```python
from build123d import *

# Parameters (mm, degrees)
F1_DEPTH  = 8
F2_W      = 15
F2_H      = 12
F2_W_2    = 4
F2_W_3    = 22
F2_W_4    = 0.5
F3_DEPTH  = 2
F4_DEPTH  = 3
F2_W_5    = 12
F2_W_6    = 2
F5_DEPTH  = 5
F6_DEPTH  = 4
F8_W      = 36.5
F8_H      = 1
F7_W      = 36.5
F7_H      = 1
F9_DEPTH  = 1
F2_H_2    = 1.5
F10_DEPTH = 3
F11_DEPTH = 2
F12_DEPTH = 2
F13_DEPTH = 3


with BuildPart() as f1:
    # F0 (on Top) → F1 (new body)
    with BuildSketch(Plane.XY):
        Polygon((-40, -7.5), (-25, -17.5), (25, -17.5), (40, -7.5), (85, -7.5), (85, 7.5), (40, 7.5), (25, 17.5), (-25, 17.5), (-40, 7.5), (-85, 7.5), (-85, -7.5), align=None)
    extrude(amount=F1_DEPTH)

    # F2 (on face) → F3 (cut)
    with BuildSketch(Plane.XY.offset(8)):
        with Locations((-77.5, 0)):
            Rectangle(F2_W, F2_H)
        with Locations((-68, 0)):
            Rectangle(F2_W_2, F2_H)
        with Locations((-55, 0)):
            Rectangle(F2_W_3, F2_H)
        with Locations((-43.75, 0)):
            Rectangle(F2_W_4, F2_H)
        with Locations((77.5, 0)):
            Rectangle(F2_W, F2_H)
        with Locations((68, 0)):
            Rectangle(F2_W_2, F2_H)
        with Locations((55, 0)):
            Rectangle(F2_W_3, F2_H)
        with Locations((43.75, 0)):
            Rectangle(F2_W_4, F2_H)
    extrude(amount=-F3_DEPTH, mode=Mode.SUBTRACT)

    # F2 (on face) → F4 (cut)
    with BuildSketch(Plane.XY.offset(8)):
        with Locations((-36, 0)):
            Rectangle(F2_W, F2_H)
        with Locations((36, 0)):
            Rectangle(F2_W, F2_H)
    extrude(amount=-F4_DEPTH, mode=Mode.SUBTRACT)

    # F2 (on face) → F5 (cut)
    with BuildSketch(Plane.XY.offset(8)):
        with Locations((-22.5, 0)):
            Rectangle(F2_W_5, F2_H)
        with Locations((-15.5, 0)):
            Rectangle(F2_W_6, F2_H)
        with Locations((15.5, 0)):
            Rectangle(F2_W_6, F2_H)
        with Locations((22.5, 0)):
            Rectangle(F2_W_5, F2_H)
    extrude(amount=-F5_DEPTH, mode=Mode.SUBTRACT)

    # F2 (on face) → F6 (cut)
    with BuildSketch(Plane.XY.offset(8)):
        Polygon((16.5, 11), (-16.5, 11), (-16.5, 6), (-14.5, 6), (-14.5, -6), (-16.5, -6), (-16.5, -11), (16.5, -11), (16.5, -6), (14.5, -6), (14.5, 6), (16.5, 6), align=None)
    extrude(amount=-F6_DEPTH, mode=Mode.SUBTRACT)

    # F8 (on face) + F7 (on face) → F9 (cut)
    with BuildSketch(Plane.XY.offset(6)):
        with Locations((61.75, 0)):
            Rectangle(F8_W, F8_H)
    with BuildSketch(Plane.XY.offset(6)):
        with Locations((-61.75, 0)):
            Rectangle(F7_W, F7_H)
    extrude(amount=-F9_DEPTH, mode=Mode.SUBTRACT)

    # F2 (on face) → F10 (cut)
    with BuildSketch(Plane.XY.offset(8)):
        with Locations((-77.5, 6.75)):
            Rectangle(F2_W, F2_H_2)
        with Locations((-77.5, 0)):
            Rectangle(F2_W, F2_H)
        with Locations((-77.5, -6.75)):
            Rectangle(F2_W, F2_H_2)
    extrude(amount=-F10_DEPTH, mode=Mode.SUBTRACT)

    # F2 (on face) → F11 (cut)
    with BuildSketch(Plane.XY.offset(8)):
        with Locations((-55, 6.75)):
            Rectangle(F2_W_3, F2_H_2)
        with Locations((-55, -6.75)):
            Rectangle(F2_W_3, F2_H_2)
    extrude(amount=-F11_DEPTH, mode=Mode.SUBTRACT)

    # F2 (on face) → F12 (cut)
    with BuildSketch(Plane.XY.offset(8)):
        with Locations((55, 6.75)):
            Rectangle(F2_W_3, F2_H_2)
        with Locations((55, -6.75)):
            Rectangle(F2_W_3, F2_H_2)
    extrude(amount=-F12_DEPTH, mode=Mode.SUBTRACT)

    # F2 (on face) → F13 (cut)
    with BuildSketch(Plane.XY.offset(8)):
        with Locations((77.5, 6.75)):
            Rectangle(F2_W, F2_H_2)
        with Locations((77.5, -6.75)):
            Rectangle(F2_W, F2_H_2)
        with Locations((77.5, 0)):
            Rectangle(F2_W, F2_H)
    extrude(amount=-F13_DEPTH, mode=Mode.SUBTRACT)


solid = f1.part
```
Geometry: final body of the model. Coordinates: model frame, mm. A direction names the side the tool comes from. Round coordinates to 2 decimals unless told otherwise and drop trailing zeros. Order: outer loops, then holes, each group sorted by start corner. A loop starts at its lowest first (then second) coordinate and runs counter-clockwise, first axis right, second up. Notation, with made-up numbers: M 50.25,-9 L 55.25,-9 A33 cw 55.25,23 Z; hole C 41,-14.75 d10. An arc over 180 degrees is marked long. Use one line per item in the form item = value. Start each with the question number.
Q1. Access query for faces 1 (the face through (-32.605, -12.43, 3.944)), 2 (the face through (63, 7.5, 3)), 3 (the face through (70, 4.83, 5.85)), 4 (the face through (29, 6, 6)). Directions: +Z, -Z, +X, -X, +Y, -Y. A direction counts if a zero-diameter tool reaches every point of the face in a straight line with its end or side. Return the directions, or none.
Q2. Pin query (flat end, axial travel): pin 1 Ø3 at (y, z) = (13, 6) entering from +X; pin 2 Ø1 at (x, z) = (34.5, 3.5) entering from +Y; pin 3 Ø0.5 at (x, z) = (56.5, 5.5) entering from -Y; pin 4 Ø6 at (x, y) = (45, -1) entering from -Z. Return the tip coordinate at first contact, or that it passes through.
Q3. Cut plane A-A (z = 1.75). Return loops of the section in (x, y).
Q4. Material intervals for line 1 (X direction, y = 5.5, z = 5.5); line 2 (Y direction, x = -1, z = 4.5); line 3 (Y direction, x = -23.5, z = 4.5), sorted ascending. Write a range as [from, to].
Q5. Cut plane B-B (y = 4.5). Return loops of the section in (x, z).
Q6. Cut plane D-D (x = 38). Return loops of the section in (y, z), and give its area (3 significant figures).
Q7. Cut plane C-C (x = 62). Return loops of the section in (y, z).
Q8. Mould query, pull axis X, two halves, no side actions, for faces 5 (the face through (-62, 7.5, 3)), 6 (the face through (-70, 4.73, 5.85)), 7 (the face through (85, 0, 2)), 8 (the face through (0, -11, 6)). Classes: +X half, -X half, draft (parallel to the pull), parting line (faces both ways), or undercut.
Geometry results:
q1.face_1 = +Z, -Z, -X, -Y
q1.face_2 = +Z, -Z, +X, +Y
q1.face_3 = +Z, +X, +Y, -Y
q1.face_4 = +Z
q2.pin_1 = 34
q2.pin_2 = 11.5
q2.pin_3 = -7.5
q2.pin_4 = 0
q3.outline = M -85,-7.5 L -40,-7.5 L -25,-17.5 L 25,-17.5 L 40,-7.5 L 85,-7.5 L 85,7.5 L 40,7.5 L 25,17.5 L -25,17.5 L -40,7.5 L -85,7.5 Z
q4.line_1 = [-70, -43.5], [43.5, 70]
q4.line_2 = [-17.5, -11], [11, 17.5]
q4.line_3 = [-17.5, -6], [6, 17.5]
q5.outline = M -85,0 L 85,0 L 85,5 L 70,5 L 70,6 L 43.5,6 L 43.5,5 L 28.5,5 L 28.5,3 L 14.5,3 L 14.5,4 L -14.5,4 L -14.5,3 L -28.5,3 L -28.5,5 L -43.5,5 L -43.5,6 L -70,6 L -70,5 L -85,5 Z
q6.outline = M -8.83,0 L 8.83,0 L 8.83,8 L 6,8 L 6,5 L -6,5 L -6,8 L -8.83,8 Z
q6.area = 105 mm^2
q7.outline = M -7.5,0 L 7.5,0 L 7.5,6 L 0.5,6 L 0.5,5 L -0.5,5 L -0.5,6 L -7.5,6 Z
q8.face_5 = draft
q8.face_6 = -X half
q8.face_7 = +X half
q8.face_8 = undercut
